```python
from build123d import *

# Parameters (mm, degrees)
SKETCH1_R           = 2.51
SKETCH1_R_2         = 2.5
SKETCH1_R_3         = 1.6
SKETCH1_R_4         = 2
BOSS_EXTRUDE1_DEPTH = 2
FILLET1_R           = 5
CUT_EXTRUDE2_DEPTH  = 47.884332404


with BuildPart() as part:
    # Sketch1 → Boss-Extrude1 (new body)
    with BuildSketch(Plane(origin=(0, 0, 0), x_dir=(1, 0, 0), z_dir=(0, 1, 0))):
        Polygon((0, 0), (26.5, 0), (26.5, -42.791666667), (0, -25.727272727), align=None)
        with Locations(Location((5, -23, 0), (0, 0, 270))):
            Circle(SKETCH1_R, mode=Mode.SUBTRACT)
        with Locations(Location((21.5, -33.625, 0), (0, 0, 270))):
            Circle(SKETCH1_R_2, mode=Mode.SUBTRACT)
        with Locations(Location((21.5, -5, 0), (0, 0, 270))):
            Circle(SKETCH1_R_3, mode=Mode.SUBTRACT)
        with Locations(Location((5, -5, 0), (0, 0, 270))):
            Circle(SKETCH1_R_3, mode=Mode.SUBTRACT)
        with Locations(Location((21.5, -13.325, 0), (0, 0, 270))):
            Circle(SKETCH1_R_4, mode=Mode.SUBTRACT)
    extrude(amount=BOSS_EXTRUDE1_DEPTH)

    # Fillet1
    fillet1_edges = [part.edges().sort_by_distance(p)[0] for p in [
        (0, 1, 0),
        (26.5, 1, 0),
        (26.5, 1, 42.791666667),
        (0, 1, 25.727272727),
    ]]
    fillet(fillet1_edges, radius=FILLET1_R)

    # Sketch2 → Cut-Extrude2 (cut, through all)
    with BuildSketch(Plane(origin=(0, 2, 0), x_dir=(1, 0, 0), z_dir=(0, 1, 0))):
        with BuildLine():
            Line((17.861538493, -32.983441068), (17.762917332, -32.966051496))
            ThreePointArc((17.762917332, -32.966051496), (17.630853466, -32.879452656), (17.602786281, -32.724042048))
            ThreePointArc((17.602786281, -32.724042048), (21.5, -29.625), (25.397213719, -32.724042048))
            ThreePointArc((25.397213719, -32.724042048), (25.369146534, -32.879452656), (25.237082668, -32.966051496))
            Line((25.237082668, -32.966051496), (25.138461507, -32.983441068))
            ThreePointArc((25.138461507, -32.983441068), (24.993487988, -32.953351583), (24.908935554, -32.831804949))
            ThreePointArc((24.908935554, -32.831804949), (23.907056069, -31.084118051), (22.107768622, -30.178172864))
            ThreePointArc((22.107768622, -30.178172864), (21.528540656, -30.583752652), (21.934120444, -31.162980617))
            ThreePointArc((21.934120444, -31.162980617), (21.5, -31.125), (21.065879556, -31.162980617))
            ThreePointArc((21.065879556, -31.162980617), (21.471459344, -30.583752652), (20.892231378, -30.178172864))
            ThreePointArc((20.892231378, -30.178172864), (19.092943931, -31.084118051), (18.091064446, -32.831804949))
            ThreePointArc((18.091064446, -32.831804949), (18.006512012, -32.953351583), (17.861538493, -32.983441068))
        make_face()
        with BuildLine():
            Line((1.361538493, -22.358441068), (1.262917332, -22.341051496))
            ThreePointArc((1.262917332, -22.341051496), (1.130853466, -22.254452656), (1.102786281, -22.099042048))
            ThreePointArc((1.102786281, -22.099042048), (5, -19), (8.897213719, -22.099042048))
            ThreePointArc((8.897213719, -22.099042048), (8.869146534, -22.254452656), (8.737082668, -22.341051496))
            Line((8.737082668, -22.341051496), (8.638461507, -22.358441068))
            ThreePointArc((8.638461507, -22.358441068), (8.493487988, -22.328351583), (8.408935554, -22.206804949))
            ThreePointArc((8.408935554, -22.206804949), (7.407056069, -20.459118051), (5.607768622, -19.553172864))
            ThreePointArc((5.607768622, -19.553172864), (5.028540656, -19.958752652), (5.434120444, -20.537980617))
            ThreePointArc((5.434120444, -20.537980617), (5, -20.5), (4.565879556, -20.537980617))
            ThreePointArc((4.565879556, -20.537980617), (4.971459344, -19.958752652), (4.392231378, -19.553172864))
            ThreePointArc((4.392231378, -19.553172864), (2.592943931, -20.459118051), (1.591064446, -22.206804949))
            ThreePointArc((1.591064446, -22.206804949), (1.506512012, -22.328351583), (1.361538493, -22.358441068))
        make_face()
    extrude(amount=-CUT_EXTRUDE2_DEPTH, mode=Mode.SUBTRACT)


solid = part.part
```
For this review, take the finished solid that the model builds, in its own axes (mm). A direction names the side the tool comes from. Round coordinates to 2 decimals unless told otherwise and drop trailing zeros. Write each loop counter-clockwise with the first axis right and the second up, starting at its lowest first coordinate (ties: lowest second). Pieces come first, ordered by that corner, then holes. Notation, with made-up numbers: M 10.5,56.5 L 53.5,56.5 A36 ccw 53.5,94.5 Z; hole C 30.25,25.25 d4. An arc over 180 degrees is marked long. One line per item, written item: value. Start each with the question number.
(1) Wall thickness on line 1 (X direction, y = 0.15, z = 5); line 2 (X direction, y = 1.65, z = 23); line 3 (Z direction, x = 2, y = 0.9): over which ranges is each line inside the solid? List them lowest first.
(2) We need section C-C (x = 3). Give the boundary of the cut face in (y, z).
(3) We need section B-B (z = 21.5). Give the boundary of the cut face in (x, y), and give its area (3 significant figures).
(4) The part is to be moulded in two halves that separate along Z. For faces 3 (the flat face through (13, 2, 19)), 4 (the flat face through (10.66, 0.99, 32.59)), 5 (the cylindrical face through (5.11, 1.01, 19.76)), say which applies: released by +Z, released by -Z, zero draft, split by the parting line, or undercut.
(5) We need section D-D (y = 1.45). Count the separate pieces of the cut face and the enclosed holes in it, and give its area (3 significant figures).
(6) Machinability: for faces 1 (the cylindrical face through (7.43, 1.01, 20.48)), 2 (the flat face through (26.5, 1, 19)), which of the approach directions +Z, -Z, +X, -X, +Y, -Y give a long, thin tool a straight path to every point of the face, cutting with its end or side? Answer none if there is none.
(7) We need section A-A (z = 35.5). Give the boundary of the cut face in (x, y), and give its area (3 significant figures).
(8) Insertion check: pin 1 (3 mm diameter, centred on x = 21.5, z = 13.325, fed in from -Y). The pin has a flat end and moves straight along its axis. Give the tip position at first contact, or say it passes through.
Result:
1. line 1: 0 to 3.4, 6.6 to 19.9, 23.1 to 26.5
1. line 2: 0 to 2.49, 7.51 to 26.5
1. line 3: 1 to 20.35, 21.2 to 27
2. outline: M 0,0.42 L 2,0.42 L 2,19.54 L 0,19.54 Z; M 0,20.13 L 2,20.13 L 2,21.48 L 0,21.48 Z; M 0,24.52 L 2,24.52 L 2,27.66 L 0,27.66 Z
3. outline: M 0,0 L 1.29,0 L 1.29,2 L 0,2 Z; M 1.84,0 L 2.99,0 L 2.99,2 L 1.84,2 Z; M 7.01,0 L 8.16,0 L 8.16,2 L 7.01,2 Z; M 8.71,0 L 26.5,0 L 26.5,2 L 8.71,2 Z
3. area: 42.8 mm²
4. face 3: zero draft
4. face 4: released by +Z
4. face 5: undercut
5. separate pieces: 1
5. enclosed holes: 5
5. area: 798 mm²
6. face 1: +Y, -Y
6. face 2: +Z, -Z, +X, +Y, -Y
7. outline: M 15.18,0 L 19.85,0 L 19.85,2 L 15.18,2 Z; M 23.15,0 L 26.14,0 L 26.14,2 L 23.15,2 Z
7. area: 15.3 mm²
8. pin 1: through
